The model under review builds one solid part; all positions refer to its coordinate system, in mm. A direction names the side the tool comes from. Round coordinates to 2 decimals unless told otherwise and drop trailing zeros.
```python
from build123d import *

# Parameters (mm, degrees)
SKETCH1_W           = 34.925
SKETCH1_H           = 34.925
BASE_EXTRUDE_DEPTH  = 19.05
SKETCH12_R          = 15.875
SKETCH12_R_2        = 14.25
CUT_EXTRUDE4_DEPTH  = 1.524
SKETCH3_R           = 1.625
CUT_EXTRUDE2_DEPTH  = 32.189426293
CIRPATTERN2_COUNT   = 4
SKETCH15_R          = 9.525
BOSS_EXTRUDE1_DEPTH = 3.175
SKETCH14_R          = 4.75
CUT_EXTRUDE6_DEPTH  = 34.223913639
CUT_EXTRUDE7_START  = -19.05
SKETCH16_R          = 6.35
CUT_EXTRUDE7_DEPTH  = 19.05


with BuildPart() as part:
    # Sketch1 → Base-Extrude (new body)
    with BuildSketch(Plane.XY):
        Rectangle(SKETCH1_W, SKETCH1_H)
    extrude(amount=BASE_EXTRUDE_DEPTH)

    # Sketch12 → Cut-Extrude4 (cut)
    with BuildSketch(Plane(origin=(-5.978518985, 12.821273311, 0), x_dir=(-1, 0, 0), z_dir=(0, 0, -1))):
        with Locations((-5.978518985, -12.821273311)):
            Circle(SKETCH12_R)
        with Locations((-5.978518985, -12.821273311)):
            Circle(SKETCH12_R_2, mode=Mode.SUBTRACT)
    extrude(amount=-CUT_EXTRUDE4_DEPTH, mode=Mode.SUBTRACT)

    # Sketch3 → Cut-Extrude2 (cut, through all)
    with BuildSketch(Plane.XY.offset(19.05)):
        with Locations((13.470384182, 13.470384182)):
            Circle(SKETCH3_R)
    cut_extrude2 = extrude(amount=-CUT_EXTRUDE2_DEPTH, mode=Mode.SUBTRACT)

    # CirPattern2: Cut-Extrude2 ×4 about axis
    cirpattern2_axis = Axis((0, 0, 0), (0, 0, 1))
    for i in range(1, CIRPATTERN2_COUNT):
        add(cut_extrude2.rotate(cirpattern2_axis, i * 360 / CIRPATTERN2_COUNT), mode=Mode.SUBTRACT)

    # Sketch10 → Hole3 (revolve, cut)
    with BuildSketch(Plane(origin=(0, 17.4625, 9.525), x_dir=(0, 0, 1), z_dir=(1, 0, 0))):
        Polygon((0, 0), (0, 7.799876674), (2.413, 6.35), (2.413, 4.826), (2.750466794, 0), align=None)
    revolve(axis=Axis((0, 21.469039452, 9.525), (0, -1, 0)), mode=Mode.SUBTRACT)

    # Sketch15 → Boss-Extrude1 (add)
    with BuildSketch(Plane.XY.offset(19.05)):
        with Locations(Location((0, 0, 0), (0, 0, 180))):
            Circle(SKETCH15_R)
    extrude(amount=BOSS_EXTRUDE1_DEPTH)

    # Sketch14 → Cut-Extrude6 (cut, through all)
    with BuildSketch(Plane(origin=(0, 0, 0), x_dir=(-1, 0, 0), z_dir=(0, 0, -1))):
        Circle(SKETCH14_R)
    extrude(amount=-CUT_EXTRUDE6_DEPTH, mode=Mode.SUBTRACT)

    # Sketch16 → Cut-Extrude7 (cut)
    with BuildSketch(Plane(origin=(0, 0, 0), x_dir=(-1, 0, 0), z_dir=(0, 0, -1)).offset(CUT_EXTRUDE7_START)):
        Circle(SKETCH16_R)
    extrude(amount=CUT_EXTRUDE7_DEPTH, mode=Mode.SUBTRACT)

    # Sketch17 → Cut-Revolve1 (revolve, cut)
    with BuildSketch(Plane(origin=(0, 0, 0), x_dir=(0, 0, -1), z_dir=(1, 0, 0))):
        Polygon((-9.525, 11.1125), (-10.514867037, 10.541), (-4.09906217, -0.5715), (-3.109195134, 0), align=None)
    revolve(axis=Axis((0, 11.1125, 9.525), (0, -0.8660254037844396, -0.4999999999999983)), mode=Mode.SUBTRACT)


solid = part.part
```
(1) To check wall thickness, follow probe 1 along Z at (x, y) = (-5.5, -9); probe 2 along Y at (x, z) = (14, 3.5); probe 3 along Y at (x, z) = (-0.5, 16). State the ranges of each line that lie inside material, in increasing order.
Data:
probe 1: z = 0 to 19.05
probe 2: y = -17.46 to -15.01, -11.93 to 11.93, 15.01 to 17.46
probe 3: y = -17.46 to -6.33, 6.33 to 17.46
(2) Consider section B-B (z = 4.5). State how many separate pieces and enclosed holes the cut face has, and give its area (3 significant figures).
Data:
separate pieces: 1
enclosed holes: 5
area: 1,060 mm2
(3) Draft analysis for pull direction Z (two halves, no side actions). For faces 4 (the flat face through (6, -3, 0)), 5 (the conical face through (-0.78, 15.08, 11.99)), 6 (the flat face through (0, -17.462, 9)), state which applies: pulls with the +Z half, pulls with the -Z half, needs draft (parallel to the pull), parting line crosses it, or undercut.
Data:
face 4: pulls with the -Z half
face 5: undercut
face 6: needs draft
(4) Insertion check: pin 1 (6 mm diameter, centred on x = 12, y = 8, fed in from +Z); pin 2 (1.9 mm diameter, centred on x = -13.47, y = 13.47, fed in from +Z); pin 3 (4.5 mm diameter, centred on x = 0, z = 9.525, fed in from +Y). Each pin has a flat end and moves straight along its axis. Give the tip position at first contact, or say it passes through.
Data:
pin 1: stops at z = 19.05
pin 2: passes through
pin 3: stops at y = 11.01
(5) For faces 1 (the cylindrical face through (-0.72, 11.89, 11.83)), 2 (the flat face through (14.2, 2.4, 1.524)), 3 (the flat face through (-8, -8, 19.05)), list the 3-axis set-ups (+Z, -Z, +X, -X, +Y, -Y) from which the entire face can be reached by the end or side of a thin tool; tool diameter is ignored.
Data:
face 1: +Y
face 2: -Z
face 3: +Z
